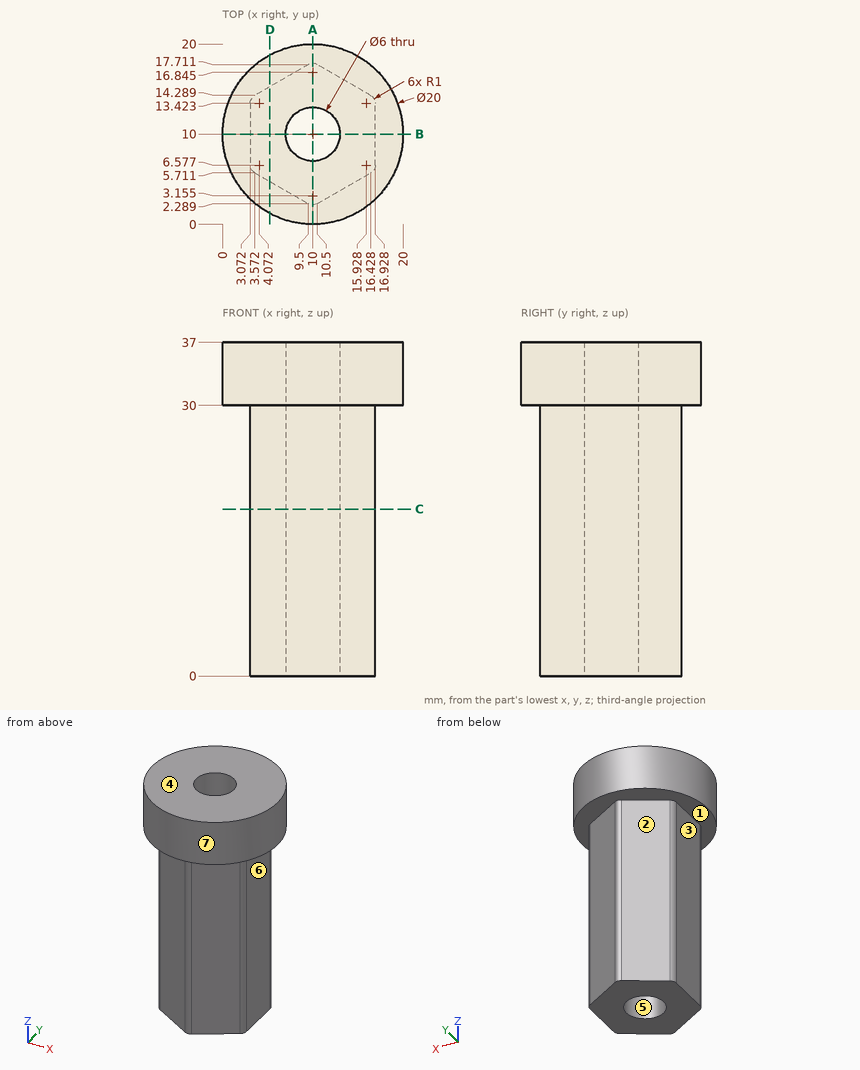
Drawing for the job (mm, zero at the part's lowest x, y, z). A direction names the side the tool comes from. Round coordinates to 2 decimals unless told otherwise and drop trailing zeros. Loops run counter-clockwise (first coordinate to the right, second up) from the corner with the lowest first, then second, coordinate; pieces in that order, holes last. Notation, with made-up numbers: (-37.75, 23.5) - (19.25, 23.5) arc R34 cw to (19.25, 58.5) - close; hole circle Ø3 at (73, -12.75). An arc over 180 degrees is marked (long way). Write each question's results on one line, items separated by ' | '.
(1) Mould opens along X. For the marked faces 4, 5, 6 and 7 say: released by +X, released by -X, zero draft, split by the parting line, or undercut.
Answer below:
face 4: zero draft | face 5: undercut | face 6: released by +X | face 7: split by the parting line
(2) Saw through at C-C, the plane z = 18.5. List the corners of the cut face in (x, y) (1 decimal).
Answer below:
outline: (3.1, 6.6) arc R1 ccw to (3.6, 5.7) - (9.5, 2.3) arc R1 ccw to (10.5, 2.3) - (16.4, 5.7) arc R1 ccw to (16.9, 6.6) - (16.9, 13.4) arc R1 ccw to (16.4, 14.3) - (10.5, 17.7) arc R1 ccw to (9.5, 17.7) - (3.6, 14.3) arc R1 ccw to (3.1, 13.4) - close; hole circle Ø6 at (10, 10)
(3) 3-axis set-ups, long thin cutter, end or side, ignore diameter. For the marked faces 1, 2 and 3: which of +Z, -Z, +X, -X, +Y, -Y reach the whole face in a straight line?
Answer below:
face 1: -Z | face 2: -Z, -X, +Y | face 3: -Z, -X, +Y, -Y
(4) Saw through at D-D, the plane x = 5.25. List the corners of the cut face in (y, z), then the cut area to 3 significant figures.
Answer below:
outline: (1.2, 30) - (4.74, 30) - (4.74, 0) - (15.26, 0) - (15.26, 30) - (18.8, 30) - (18.8, 37) - (1.2, 37) - close | area: 439 mm^2
(5) Pin check, flat tips, straight feed: pin 1 (10 mm diameter, centred on x = 13, z = 28.5, fed in from -Y); pin 2 (5.5 mm diameter, centred on y = 9.5, z = 20.5, fed in from -X); pin 3 (1.5 mm diameter, centred on x = 14.5, z = 13.5, fed in from +Y) (1 decimal); pin 4 (7.5 mm diameter, centred on y = 11, z = 9.5, fed in from +X). Stop position of each tip, or through.
Answer below:
pin 1: stops at y = 0 | pin 2: stops at x = 3.07 | pin 3: stops at y = 15.8 | pin 4: stops at x = 16.93
(6) Wall check: L1, parallel to X at y = 10, z = 13.5; L2, parallel to Z at x = 14.25, y = 17.25; L3, parallel to Y at x = 9, z = 20. Give the ranges that are in metal, low to high.
Answer below:
L1: x = 3.07 to 7, 13 to 16.93 | L2: z = 30 to 37 | L3: y = 2.58 to 7.17, 12.83 to 17.42
(7) Saw through at B-B, the plane y = 10. List the corners of the cut face in (x, z).
Answer below:
outline: (0, 30) - (3.07, 30) - (3.07, 0) - (7, 0) - (7, 37) - (0, 37) - close; (13, 0) - (16.93, 0) - (16.93, 30) - (20, 30) - (20, 37) - (13, 37) - close
(8) Saw through at A-A, the plane x = 10. List the corners of the cut face in (y, z) (1 decimal).
Answer below:
outline: (0, 30) - (2.2, 30) - (2.2, 0) - (7, 0) - (7, 37) - (0, 37) - close; (13, 0) - (17.8, 0) - (17.8, 30) - (20, 30) - (20, 37) - (13, 37) - close
